Can you work these out from the model? Positions are in its coordinate system, mm. Face numbers are marked on the shaded views. A direction names the side the tool comes from. Give positions to 0.01 mm unless a question says otherwise; leave off trailing zeros. Write each loop counter-clockwise with the first axis right and the second up, starting at its lowest first coordinate (ties: lowest second). Pieces come first, ordered by that corner, then holes. Notation, with made-up numbers: M 52,15.25 L 66,15.25 A10 ccw 66,28.25 Z; hole C 63,-27.75 d8. An arc over 180 degrees is marked long. Answer as CSV lines item,"result". Start each with the question number.
```python
from build123d import *

# Parameters (mm, degrees)
SKETCH_R  = 1.65
PAD_DEPTH = 1.6


with BuildPart() as part:
    # Sketch → Pad (new body)
    with BuildSketch(Plane.XY):
        Polygon((3.5, 5), (3.5, -22), (-3.5, -22), (-3.5, -5), (-10, -5), (-10, 5), align=None)
        Circle(SKETCH_R, mode=Mode.SUBTRACT)
        with Locations((0, -10)):
            Circle(SKETCH_R, mode=Mode.SUBTRACT)
        with Locations((0, -17.5)):
            Circle(SKETCH_R, mode=Mode.SUBTRACT)
    extrude(amount=PAD_DEPTH)


solid = part.part
```
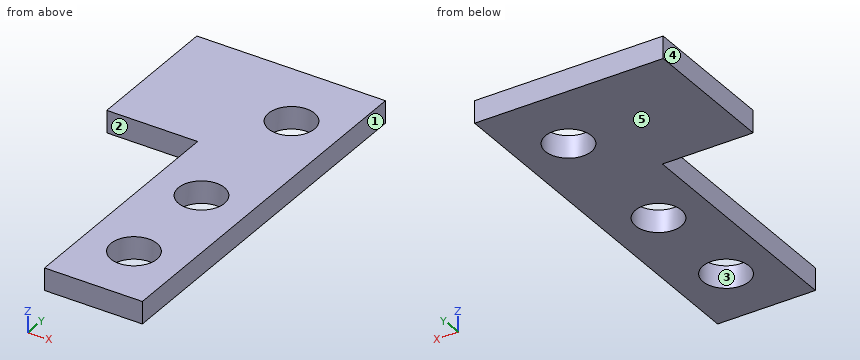
1) I want a section at D-D, the plane y = -10. Please give me the cut outline in (x, z).
2) I'm going to push a flat-ended pin straight in: P1, Ø0.5, axis at x = -5.5, z = 1, coming from the -Y side. Where does the tip first touch, or does it pass through?
3) Thinking about a two-plate mould opening in X: for the marked faces 3, 4 and 5, which applies, released by +X, released by -X, zero draft, split by the parting line, or undercut?
4) I want a section at B-B, the plane x = 0. Please give me the cut outline in (y, z).
5) I want a section at A-A, the plane y = 0. Please give me the cut outline in (x, z), then the cut area to 3 significant figures.
6) I need wall thicknesses on L1, parallel to Y at x = 0, z = 0.45; L2, parallel to X at y = -14.75, z = 1; L3, parallel to Y at x = -1.25, z = 1.1. Which ranges of each line are inside material? Lowest first, please. Write a range as from..to.
7) I want a section at C-C, the plane z = 0.3. Please give me the cut outline in (x, y), then the cut area to 3 significant figures.
8) On a 3-axis mill with a long thin cutter (end or side, diameter ignored), from which of +Z, -Z, +X, -X, +Y, -Y can I reach the whole of each face in a straight line? I mean the marked faces 1 and 2. Say none if no direction works.
Values found:
1,outline,"M -3.5,0 L -1.65,0 L -1.65,1.6 L -3.5,1.6 Z; M 1.65,0 L 3.5,0 L 3.5,1.6 L 1.65,1.6 Z"
2,P1,"stops at y = -5"
3,face 3,"undercut"
3,face 4,"released by -X"
3,face 5,"zero draft"
4,outline,"M -22,0 L -19.15,0 L -19.15,1.6 L -22,1.6 Z; M -15.85,0 L -11.65,0 L -11.65,1.6 L -15.85,1.6 Z; M -8.35,0 L -1.65,0 L -1.65,1.6 L -8.35,1.6 Z; M 1.65,0 L 5,0 L 5,1.6 L 1.65,1.6 Z"
5,outline,"M -10,0 L -1.65,0 L -1.65,1.6 L -10,1.6 Z; M 1.65,0 L 3.5,0 L 3.5,1.6 L 1.65,1.6 Z"
5,area,"16.3 mm²"
6,L1,"y = -22..-19.15, -15.85..-11.65, -8.35..-1.65, 1.65..5"
6,L2,"x = -3.5..3.5"
6,L3,"y = -22..-18.58, -16.42..-11.08, -8.92..-1.08, 1.08..5"
7,outline,"M -10,-5 L -3.5,-5 L -3.5,-22 L 3.5,-22 L 3.5,5 L -10,5 Z; hole C 0,-17.5 d3.3; hole C 0,-10 d3.3; hole C 0,0 d3.3"
7,area,"228 mm²"
8,face 1,"+Z, -Z, +X, +Y, -Y"
8,face 2,"+Z, -Z, -X, -Y"
